from build123d import *

# Parameters (mm, degrees)
F0_W     = 10
F0_H     = 120
F0_R     = 1.6
F1_DEPTH = 5
F2_R     = 4.99999
F3_R     = 1


# Not quite as in the source:
# - a fillet or chamfer is up to 0.001 mm smaller than in the source, because OpenCascade refuses the exact size


with BuildPart() as f1:
    # F0 (on Right) → F1 (new body)
    with BuildSketch(Plane.YZ):
        with Locations((0, 60)):
            Rectangle(F0_W, F0_H)
        with Locations((0, 5)):
            Circle(F0_R, mode=Mode.SUBTRACT)
        with Locations((0, 20)):
            Circle(F0_R, mode=Mode.SUBTRACT)
        with Locations((0, 30)):
            Circle(F0_R, mode=Mode.SUBTRACT)
        with Locations((0, 107)):
            Circle(F0_R, mode=Mode.SUBTRACT)
        with Locations((0, 115)):
            Circle(F0_R, mode=Mode.SUBTRACT)
    extrude(amount=F1_DEPTH)

    # F2 (radius 5 in the source; OpenCascade refuses exactly that, so slightly less here)
    f2_edges = [f1.edges().sort_by_distance(p)[0] for p in [
        (2.5, 5, 0),
        (2.5, -5, 0),
        (2.5, 5, 120),
        (2.5, -5, 120),
    ]]
    fillet(f2_edges, radius=F2_R)

    # F3
    f3_edges = [f1.edges().sort_by_distance(p)[0] for p in [
        (5, -3.535537, 118.535537),
        (0, 5, 60),
    ]]
    fillet(f3_edges, radius=F3_R)


solid = f1.part
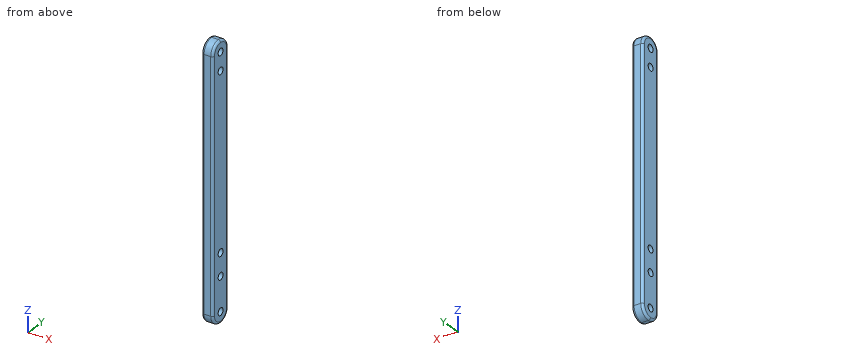
Read the model definition and answer for the solid it produces. Units are mm, in the model's axes. Round coordinates to 2 decimals unless told otherwise and drop trailing zeros. Loops run counter-clockwise (first coordinate to the right, second up) from the corner with the lowest first, then second, coordinate; pieces in that order, holes last. Notation, with made-up numbers: (47, -17.5) - (104, -17.5) arc R17 ccw to (104, 7.5) - close; hole circle Ø3 at (19.25, -28.5). An arc over 180 degrees is marked (long way). One line per question, with ' | ' between items. Start each with the question number.
Q1. Section C-C on z = 55.5 is taken. Give the vertices of the cut face in (x, y), plus the area to 3 significant figures.
Q2. Section A-A on z = 30 is taken. Give the vertices of the cut face in (x, y), plus the area to 3 significant figures.
Q3. Section B-B on x = 3.25 is taken. Count the separate pieces of the cut face and the enclosed holes in it, plus the area to 3 significant figures.
Q4. Find the intervals of material crossed by L1, parallel to Z at x = 1.75, y = 0; L2, parallel to Z at x = 4.1, y = 0.5; L3, parallel to Y at x = 2.6, z = 115, in increasing order.
Q5. Flat-ended cylindrical pins translate along their axes: pin 1 (3 mm diameter, centred on y = 0, z = 20, fed in from -X); pin 2 (1.5 mm diameter, centred on x = 1, y = -2.5, fed in from -Z); pin 3 (1 mm diameter, centred on x = 4, y = 2, fed in from +Z). Find the tip coordinate at first contact, or state that the pin passes through.
Established:
1) outline: (0, -4) arc R1 ccw to (1, -5) - (4, -5) arc R1 ccw to (5, -4) - (5, 4) arc R1 ccw to (4, 5) - (1, 5) arc R1 ccw to (0, 4) - close | area: 49.1 mm²
2) outline: (0, -4) arc R1 ccw to (1, -5) - (4, -5) arc R1 ccw to (5, -4) - (5, -1.6) - (0, -1.6) - close; (0, 1.6) - (5, 1.6) - (5, 4) arc R1 ccw to (4, 5) - (1, 5) arc R1 ccw to (0, 4) - close | area: 33.1 mm²
3) separate pieces: 1 | enclosed holes: 5 | area: 1,140 mm²
4) L1: 0 to 3.4, 6.6 to 18.4, 21.6 to 28.4, 31.6 to 105.4, 108.6 to 113.4, 116.6 to 120 | L2: 0.03 to 3.48, 6.52 to 18.48, 21.52 to 28.48, 31.52 to 105.48, 108.52 to 113.48, 116.52 to 119.97 | L3: -5 to -1.6, 1.6 to 5
5) pin 1: through | pin 2: z = 0.32 | pin 3: z = 119.77
